Can you work these out from the model? Positions are in its coordinate system, mm. A direction names the side the tool comes from. Give positions to 0.01 mm unless a question says otherwise; leave off trailing zeros. Loops run counter-clockwise (first coordinate to the right, second up) from the corner with the lowest first, then second, coordinate; pieces in that order, holes last. Notation, with made-up numbers: (49.25, -15.5) - (87.25, -15.5) arc R20 cw to (87.25, 19.5) - close; hole circle Ø6 at (-38.75, 30.25). An arc over 180 degrees is marked (long way). Answer as a JSON object with one key per item and string values.
```python
from build123d import *

# Parameters (mm, degrees)
SKETCH1_W                     = 15
SKETCH1_H                     = 23
BASE_FLANGE1_DEPTH            = 1
EDGE_FLANGE1_STRIP_W          = 4.6
EDGE_FLANGE1_STRIP_H          = 1
EDGE_FLANGE1_STRIP_CUT_DEPTH  = 23
EDGE_FLANGE1_DEPTH            = 23
SKETCH10_W                    = 10
SKETCH10_H                    = 47.7
BOSS_EXTRUDE2_DEPTH           = 1
SKETCH15_W                    = 1
SKETCH15_H                    = 34.3
BOSS_EXTRUDE3_DEPTH           = 9
EDGE_FLANGE3_STRIP_W          = 5.4732
EDGE_FLANGE3_STRIP_H          = 1
EDGE_FLANGE3_STRIP_CUT_DEPTH  = 34.3
EDGE_FLANGE3_DEPTH            = 34.3
EDGE_FLANGE4_STRIP_W          = 5.4732
EDGE_FLANGE4_STRIP_H          = 1
EDGE_FLANGE4_STRIP_CUT_DEPTH  = 7
EDGE_FLANGE4_RELIEF_W         = 5.9732
EDGE_FLANGE4_RELIEF_H         = 1000
EDGE_FLANGE4_RELIEF_CUT_DEPTH = 1
EDGE_FLANGE4_DEPTH            = 7
SKETCH31_R                    = 1.5
CUT_EXTRUDE1_DEPTH            = 82.639451248
SKETCH32_R                    = 1.5
CUT_EXTRUDE2_DEPTH            = 10


# Sheet-metal steps are written as plain solids
with BuildPart() as part:
    # Sketch1 → Base-Flange1 (new body)
    with BuildSketch(Plane(origin=(0, 0, 0), x_dir=(1, 0, 0), z_dir=(0, 1, 0))):
        with Locations((-7.5, -11.5)):
            Rectangle(SKETCH1_W, SKETCH1_H)
    extrude(amount=-BASE_FLANGE1_DEPTH)

    # Edge-Flange1 strip (across the edge) → Edge-Flange1 strip cut (cut)
    with BuildSketch(Plane(origin=(-15, -1, 23), x_dir=(1, 0, 0), z_dir=(0, 0, -1))):
        with Locations((-1, -0.5)):
            Rectangle(EDGE_FLANGE1_STRIP_W, EDGE_FLANGE1_STRIP_H)
    extrude(amount=EDGE_FLANGE1_STRIP_CUT_DEPTH, mode=Mode.SUBTRACT)

    # Edge-Flange1 section (across the edge) → Edge-Flange1 (add)
    with BuildSketch(Plane(origin=(-15, -1, 23), x_dir=(1, 0, 0), z_dir=(0, 0, -1))):
        with BuildLine():
            Line((0, 0.3), (0, 48))
            Line((0, 48), (1, 48))
            Line((1, 48), (1, 0.3))
            ThreePointArc((1, 0.3), (1.087867966, 0.087867966), (1.3, 0))
            Line((1.3, 0), (1.3, -1))
            ThreePointArc((1.3, -1), (0.380761184, -0.619238816), (0, 0.3))
        make_face()
    extrude(amount=EDGE_FLANGE1_DEPTH)

    # Sketch10 → Boss-Extrude2 (add)
    with BuildSketch(Plane.ZY.offset(15)):
        with Locations((-5, -25.15)):
            Rectangle(SKETCH10_W, SKETCH10_H)
    extrude(amount=-BOSS_EXTRUDE2_DEPTH)

    # Sketch15 → Boss-Extrude3 (add)
    with BuildSketch(Plane.XY.offset(23)):
        with Locations((-14.5, -31.85)):
            Rectangle(SKETCH15_W, SKETCH15_H)
    extrude(amount=BOSS_EXTRUDE3_DEPTH)

    # Edge-Flange3 strip (across the edge) → Edge-Flange3 strip cut (cut)
    with BuildSketch(Plane(origin=(-14, -14.7, 32), x_dir=(0, 0, -1), z_dir=(0, -1, 0))):
        with Locations((-1, -0.5)):
            Rectangle(EDGE_FLANGE3_STRIP_W, EDGE_FLANGE3_STRIP_H)
    extrude(amount=EDGE_FLANGE3_STRIP_CUT_DEPTH, mode=Mode.SUBTRACT)

    # Edge-Flange3 section (across the edge) → Edge-Flange3 (add)
    with BuildSketch(Plane(origin=(-14, -14.7, 32), x_dir=(0, 0, -1), z_dir=(0, -1, 0))):
        with BuildLine():
            Line((0, 0.7366), (0, 64))
            Line((0, 64), (1, 64))
            Line((1, 64), (1, 0.7366))
            ThreePointArc((1, 0.7366), (1.215745145, 0.215745145), (1.7366, 0))
            Line((1.7366, 0), (1.7366, -1))
            ThreePointArc((1.7366, -1), (0.508638364, -0.491361636), (0, 0.7366))
        make_face()
    extrude(amount=EDGE_FLANGE3_DEPTH)

    # Edge-Flange4 strip (across the edge) → Edge-Flange4 strip cut (cut)
    with BuildSketch(Plane(origin=(50, -42, 31), x_dir=(-1, 0, 0), z_dir=(0, -1, 0))):
        with Locations((-1, -0.5)):
            Rectangle(EDGE_FLANGE4_STRIP_W, EDGE_FLANGE4_STRIP_H)
    extrude(amount=EDGE_FLANGE4_STRIP_CUT_DEPTH, mode=Mode.SUBTRACT)

    # Edge-Flange4 relief (on the sheet) → Edge-Flange4 relief cut (cut)
    with BuildSketch(Plane(origin=(48.2634, -42, 31), x_dir=(-1, 0, 0), z_dir=(0, 0, -1))):
        with Locations((-2.4866, 500)):
            Rectangle(EDGE_FLANGE4_RELIEF_W, EDGE_FLANGE4_RELIEF_H)
    extrude(amount=-EDGE_FLANGE4_RELIEF_CUT_DEPTH, mode=Mode.SUBTRACT)

    # Edge-Flange4 section (across the edge) → Edge-Flange4 (add)
    with BuildSketch(Plane(origin=(50, -42, 31), x_dir=(-1, 0, 0), z_dir=(0, -1, 0))):
        with BuildLine():
            Line((0, 0.7366), (0, 7.5))
            Line((0, 7.5), (1, 7.5))
            Line((1, 7.5), (1, 0.7366))
            ThreePointArc((1, 0.7366), (1.215745145, 0.215745145), (1.7366, 0))
            Line((1.7366, 0), (1.7366, -1))
            ThreePointArc((1.7366, -1), (0.508638364, -0.491361636), (0, 0.7366))
        make_face()
    extrude(amount=EDGE_FLANGE4_DEPTH)

    # Sketch31 → Cut-Extrude1 (cut, through all)
    with BuildSketch(Plane.XY.offset(32)):
        with Locations((3, -40)):
            Circle(SKETCH31_R)
        with Locations((13, -22.5)):
            Circle(SKETCH31_R)
    extrude(amount=-CUT_EXTRUDE1_DEPTH, mode=Mode.SUBTRACT)

    # Sketch32 → Cut-Extrude2 (cut)
    with BuildSketch(Plane(origin=(0, 0, 0), x_dir=(1, 0, 0), z_dir=(0, 1, 0))):
        with Locations(Location((-6, -4, 0), (0, 0, 270))):
            Circle(SKETCH32_R)
        with Locations(Location((-6, -19, 0), (0, 0, 270))):
            Circle(SKETCH32_R)
    extrude(amount=-CUT_EXTRUDE2_DEPTH, mode=Mode.SUBTRACT)


solid = part.part
```
1) Imagine slicing it at C-C on x = 13. Write out the boundary of the cut face in (y, z), and give its area (3 significant figures).
Check sheet entries:
{"outline": "(-49, 31) - (-24, 31) - (-24, 32) - (-49, 32) - close; (-21, 31) - (-14.7, 31) - (-14.7, 32) - (-21, 32) - close", "area": "31.3 mm2"}
2) Imagine slicing it at B-B on y = -22.5. Write out the boundary of the cut face in (x, z).
Check sheet entries:
{"outline": "(-15, -10) - (-14, -10) - (-14, 30.26) arc R0.74 cw to (-13.26, 31) - (11.5, 31) - (11.5, 32) - (-13.26, 32) arc R1.74 ccw to (-15, 30.26) - close; (14.5, 31) - (47.76, 31) - (47.76, 32) - (14.5, 32) - close"}
3) I'm going to push flat-ended pins straight in: P1, Ø5, axis at y = -22.5, z = 12, coming from the +X side; P2, Ø7, axis at x = -5, z = 7.5, coming from the -Y side; P3, Ø0.8, axis at x = 49.5, y = -47, coming from the -Z side. Where does each tip first touch, or does it pass through?
Check sheet entries:
{"P1": "x = -14", "P2": "y = -1", "P3": "z = 23.5"}
4) I need wall thicknesses on L1, parallel to X at y = -42.5, z = 29; L2, parallel to X at y = -32.5, z = 25.5; L3, parallel to Z at x = 19.5, y = -22.5. Which ranges of each line are inside material? Lowest first, please.
Check sheet entries:
{"L1": "-15 to -14, 49 to 50", "L2": "-15 to -14", "L3": "31 to 32"}
5) Imagine slicing it at D-D on y = -32. Write out the boundary of the cut face in (x, z).
Check sheet entries:
{"outline": "(-15, -10) - (-14, -10) - (-14, 30.26) arc R0.74 cw to (-13.26, 31) - (47.76, 31) - (47.76, 32) - (-13.26, 32) arc R1.74 ccw to (-15, 30.26) - close"}
6) Which directions (+Z, -Z, +X, -X, +Y, -Y) give clear straight access to the entire face, cutting with the end or side of a thin tool? Please do faces 4 (the flat face through (49, -45, 27)), 5 (the flat face through (49.4, -42, 27.7)), 6 (the flat face through (-7, -1, 11)).
Check sheet entries:
{"face 4": "-Z, +Y, -Y", "face 5": "+Z, -Z, +X, +Y", "face 6": "+Z, -Z, +X, -Y"}
7) If we mould it in two halves opening along Z, with no side actions, what happens to faces 1 (the cylindrical face through (-5.93, -0.49, 17.5)), 2 (the flat face through (-10.24, -0.85, 23)), 3 (the flat face through (50, -45, 27))? For each: released by +Z, released by -Z, zero draft, split by the parting line, or undercut.
Check sheet entries:
{"face 1": "undercut", "face 2": "released by +Z", "face 3": "zero draft"}
8) Imagine slicing it at A-A on z = 19. Write out the boundary of the cut face in (x, y), and give its area (3 significant figures).
Check sheet entries:
{"outline": "(-15, -49) - (-14, -49) - (-14, -1.3) arc R0.3 cw to (-13.7, -1) - (-7.5, -1) - (-7.5, 0) - (-13.7, 0) arc R1.3 ccw to (-15, -1.3) - close; (-4.5, -1) - (0, -1) - (0, 0) - (-4.5, 0) - close", "area": "59.7 mm2"}
